Can you work these out from the drawing? Everything is in mm from the part's minimum corner. Round coordinates to 2 decimals unless told otherwise and drop trailing zeros. Loops run counter-clockwise (first coordinate to the right, second up) from the corner with the lowest first, then second, coordinate; pieces in that order, holes last. Notation, with made-up numbers: (78.5, 76.5) -> (96.5, 76.5) arc R19 ccw to (96.5, 109.5) -> close; hole circle Ø4 at (-16.75, 33). An arc over 180 degrees is marked (long way). One line per item, written item: value.
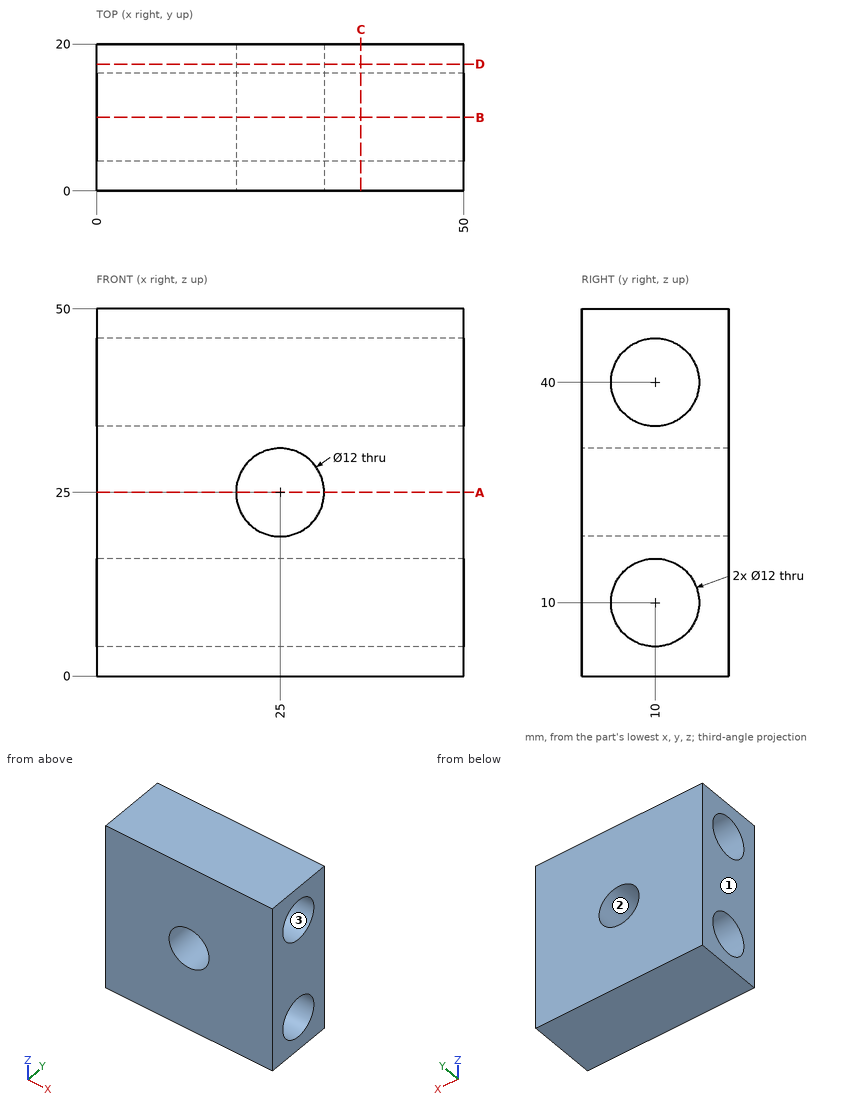
(1) If we section it at A-A, the plane z = 25: Please give me the cut outline in (x, y), then the cut area to 3 significant figures.
Recorded:
outline: (0, 0) -> (19, 0) -> (19, 20) -> (0, 20) -> close; (31, 0) -> (50, 0) -> (50, 20) -> (31, 20) -> close
area: 760 mm²
(2) If we section it at C-C, the plane x = 36: Please give me the cut outline in (y, z), then the cut area to 3 significant figures.
Recorded:
outline: (0, 0) -> (20, 0) -> (20, 50) -> (0, 50) -> close; hole circle Ø12 at (10, 10); hole circle Ø12 at (10, 40)
area: 774 mm²
(3) Thinking about a two-plate mould opening in X: for the marked faces 1, 2 and 3, which applies, released by +X, released by -X, zero draft, split by the parting line, or undercut?
Recorded:
face 1: released by -X
face 2: undercut
face 3: zero draft
(4) If we section it at B-B, the plane y = 10: Please give me the cut outline in (x, z).
Recorded:
outline: (0, 0) -> (50, 0) -> (50, 4) -> (0, 4) -> close; (0, 16) -> (50, 16) -> (50, 34) -> (0, 34) -> close; (0, 46) -> (50, 46) -> (50, 50) -> (0, 50) -> close; hole circle Ø12 at (25, 25)
(5) If I drill on L1, parallel to Z at x = 12, y = 10; L2, parallel to Z at x = 37, y = 13.5; L3, parallel to Y at x = 17.5, z = 10, over which ranges is the centre line in solid material (lowest first)?
Recorded:
L1: 0 to 4, 16 to 34, 46 to 50
L2: 0 to 5.13, 14.87 to 35.13, 44.87 to 50
L3: 0 to 4, 16 to 20
(6) If we section it at D-D, the plane y = 17.25: Please give me the cut outline in (x, z), then the cut area to 3 significant figures.
Recorded:
outline: (0, 0) -> (50, 0) -> (50, 50) -> (0, 50) -> close; hole circle Ø12 at (25, 25)
area: 2,390 mm²
